Geometry: final body of the model. Coordinates: model frame, mm. Coordinates: 2 decimals unless noted, no trailing zeros. Write each loop counter-clockwise with the first axis right and the second up, starting at its lowest first coordinate (ties: lowest second). Pieces come first, ordered by that corner, then holes. Notation, with made-up numbers: (-37.5, -5.5) - (2.5, -5.5) arc R19 cw to (2.5, -1.5) - close; hole circle Ø2 at (71, 75). An arc over 180 degrees is marked (long way). Answer as a JSON object with one key per item and string values. Group by question number.
Item 1: Section B-B on x = -40. Return loops of the section in (y, z), and give its area (3 significant figures).
Item 2: Section A-A on y = -10. Return loops of the section in (x, z), and give its area (3 significant figures).
Item 3: Line query: line 1 along Y through (x, z) = (-40, 2.75); line 2 along X through (y, z) = (9.25, -3.5); line 3 along X through (y, z) = (-8.75, -1.5). Output: solid intervals per line, ascending. Write a range as from..to.
Item 4: Mould query, pull axis Y, two halves, no side actions, for faces 1 (the flat face through (-1, -15, 0)), 2 (the cylindrical face through (-39.169, -11.597, 0.07)), 3 (the flat face through (-1, 0, -5)). Classes: pulls with the +Y half, pulls with the -Y half, needs draft (parallel to the pull), parting line crosses it, or undercut.
```python
from build123d import *

# Parameters (mm, degrees)
F0_W     = 90
F0_H     = 30
F1_DEPTH = 5
F2_R     = 1.8
F3_DEPTH = 21
F4_R     = 1.8
F5_DEPTH = 21


with BuildPart() as f1:
    # F0 (on Top) → F1 (new body, symmetric)
    with BuildSketch(Plane.XY):
        Rectangle(F0_W, F0_H)
    extrude(amount=F1_DEPTH, both=True)

    # F2 (on face) → F3 (cut)
    with BuildSketch(Plane.XY.offset(5)):
        with Locations((-40, 10)):
            Circle(F2_R)
    extrude(amount=-F3_DEPTH, mode=Mode.SUBTRACT)

    # F4 (on face) → F5 (cut)
    with BuildSketch(Plane.XY.offset(5)):
        with Locations((-40, -10)):
            Circle(F4_R)
    extrude(amount=-F5_DEPTH, mode=Mode.SUBTRACT)


solid = f1.part
```
Checks:
{
 "1": {"outline": "(-15, -5) - (-11.8, -5) - (-11.8, 5) - (-15, 5) - close; (-8.2, -5) - (8.2, -5) - (8.2, 5) - (-8.2, 5) - close; (11.8, -5) - (15, -5) - (15, 5) - (11.8, 5) - close", "area": "228 mm^2"},
 "2": {"outline": "(-45, -5) - (-41.8, -5) - (-41.8, 5) - (-45, 5) - close; (-38.2, -5) - (45, -5) - (45, 5) - (-38.2, 5) - close", "area": "864 mm^2"},
 "3": {"line 1": "-15..-11.8, -8.2..8.2, 11.8..15", "line 2": "-45..-41.64, -38.36..45", "line 3": "-45..-41.3, -38.7..45"},
 "4": {"face 1": "pulls with the -Y half", "face 2": "undercut", "face 3": "needs draft"}
}
